```python
from build123d import *

# Parameters (mm, degrees)
F0_R           = 30
F1_DEPTH       = 58
F2_R           = 60
F2_R_2         = 30
F3_DEPTH       = 15
F4_R           = 18.475
F5_DEPTH       = 12.5
F6_D           = 6.6
F6_CBORE_D     = 11.25
F6_CBORE_DEPTH = 6
F7_R           = 20.975
F8_DEPTH       = 12
F10_D          = 28.9
F11_SIZE       = 1


# Not quite as in the source:
# - a feature names something its author has since deleted; it is built from what else it names


with BuildPart() as f1:
    # F0 (on Top) → F1 (new body)
    with BuildSketch(Plane.XY):
        Circle(F0_R)
    extrude(amount=F1_DEPTH)

    # F2 (on face) → F3 (join)
    with BuildSketch(Plane.XY.offset(58)):
        Circle(F2_R)
        Circle(F2_R_2, mode=Mode.SUBTRACT)
        Circle(F2_R_2)
    extrude(amount=F3_DEPTH)

    # F4 (on face) → F5 (cut)
    with BuildSketch(Plane.XY.offset(73)):
        Circle(F4_R)
    extrude(amount=-F5_DEPTH, mode=Mode.SUBTRACT)

    # F6 (through all)
    with Locations(Plane.XY.offset(73)):
        with Locations((-43.3012701892, -25), (0, 50), (43.3012701892, -25)):
            CounterBoreHole(F6_D / 2, F6_CBORE_D / 2, F6_CBORE_DEPTH)

    # F7 (on face) → F8 (cut)
    with BuildSketch(Plane(origin=(0, 0, 0), x_dir=(1, 0, 0), z_dir=(0, 0, -1))):
        Circle(F7_R)
    extrude(amount=-F8_DEPTH, mode=Mode.SUBTRACT)

    # F10 (through all)
    with Locations(Plane.XY.offset(73)):
        with Locations((0, 0)):
            Hole(F10_D / 2)

    # F11
    f11_edges = [f1.edges().sort_by_distance(p)[0] for p in [
        (-60, 0, 73),
        (-60, 0, 58),
        (-30, 0, 0),
        (-20.975, 0, 0),
        (-18.475, 0, 73),
    ]]
    chamfer(f11_edges, length=F11_SIZE)


solid = f1.part
```
Here's how the part is built. I have some questions about the finished solid (model axes, mm). A direction names the side the tool comes from. Coordinates: 2 decimals unless noted, no trailing zeros. Order: outer loops, then holes, each group sorted by start corner. A loop starts at its lowest first (then second) coordinate and runs counter-clockwise, first axis right, second up. Notation, with made-up numbers: (-2, 28) -> (30, 28) arc R24 ccw to (30, 53) -> close; hole circle Ø11 at (-35, 64). An arc over 180 degrees is marked (long way). Return JSON: item names as keys, results as strings.
1) If we section it at B-B on x = 0: State how many separate pieces and enclosed holes the cut face has, plus the area to 3 significant figures.
Conclusion:
{"separate pieces": "3", "enclosed holes": "0", "area": "2,780 mm²"}
2) Thinking about a two-plate mould opening in X: for faces 4 (the cylindrical face through (40.25, -26.26, 62.44)), 5 (the flat face through (0, 46, 67)), 6 (the cylindrical face through (-29.97, 1.32, 29.1)), 7 (the flat face through (-4, 22, 0)), which applies, +X half, -X half, draft (parallel to the pull), parting line (faces both ways), or undercut?
Conclusion:
{"face 4": "undercut", "face 5": "undercut", "face 6": "parting line", "face 7": "draft"}
3) If we section it at A-A on z = 34: List the corners of the cut face in (x, y) for me.
Conclusion:
{"outline": "circle Ø60 at (0, 0); hole circle Ø28.9 at (0, 0)"}
4) If I drill on probe 1 along Y at (x, z) = (0, 7) (3 decimals); probe 2 along X at (y, z) = (14, 65.5); probe 3 along Z at (x, y) = (14, -44.5), over which ranges is the centre line in solid material (lowest first)?
Conclusion:
{"probe 1": "y = -30 to -20.975, 20.975 to 30", "probe 2": "x = -58.34 to -12.06, 12.06 to 58.34", "probe 3": "z = 58 to 73"}
5) On a 3-axis mill with a long thin cutter (end or side, diameter ignored), from which of +Z, -Z, +X, -X, +Y, -Y can I reach the whole of each face in a straight line? I mean faces 1 (the cylindrical face through (-59.94, 2.64, 65.41)), 2 (the cylindrical face through (-4.005, -18.036, 66.33)), 3 (the flat face through (-14, 27, 58)). Say none if no direction works.
Conclusion:
{"face 1": "+Z, -Z", "face 2": "+Z", "face 3": "-Z"}
6) I'm going to push flat-ended pins straight in: P1, Ø8.5, axis at x = 43.3, y = -25, coming from the -Z side; P2, Ø6, axis at x = 18, z = 42, coming from the +Y side; P3, Ø6, axis at x = 42.5, z = 52.5, coming from the -Y side; P4, Ø21, axis at x = -3, y = 10, coming from the -Z side. Where does each tip first touch, or does it pass through?
Conclusion:
{"P1": "stops at z = 58", "P2": "stops at y = 25.98", "P3": "passes through", "P4": "stops at z = 12"}
